```python
from build123d import *

# Parameters (mm, degrees)
SKETCH_1_R      = 1.55
EXTRUDE_1_DEPTH = 3
FILLET_1_R      = 2


with BuildPart() as part:
    # 草图1 → 凸台-拉伸1 (new body)
    with BuildSketch(Plane(origin=(0, 0, 0), x_dir=(0, 0, -1), z_dir=(1, 0, 0))):
        with BuildLine():
            Line((0, 25.4), (0, 0))
            Line((0, 0), (17, 0))
            Line((17, 0), (17, 33))
            Line((17, 33), (-5.5, 33))
            Line((-5.5, 33), (0, 27.5))
            ThreePointArc((0, 27.5), (0.74246212, 27.19246212), (1.05, 26.45))
            ThreePointArc((1.05, 26.45), (0.74246212, 25.70753788), (0, 25.4))
        make_face()
        with Locations((7.75, 5)):
            Circle(SKETCH_1_R, mode=Mode.SUBTRACT)
        with Locations((2.5, 29)):
            Circle(SKETCH_1_R, mode=Mode.SUBTRACT)
        with Locations((7.75, 20)):
            Circle(SKETCH_1_R, mode=Mode.SUBTRACT)
        with Locations((13, 29)):
            Circle(SKETCH_1_R, mode=Mode.SUBTRACT)
    extrude(amount=EXTRUDE_1_DEPTH)

    # 圆角1
    fillet_1_edges = [part.edges().sort_by_distance(p)[0] for p in [
        (1.5, 33, 5.5),
    ]]
    fillet(fillet_1_edges, radius=FILLET_1_R)


solid = part.part
```
The listing builds one solid part. Answer for the finished solid, in the listing's coordinates (mm). A direction names the side the tool comes from. Give positions to 0.01 mm unless a question says otherwise; leave off trailing zeros. Order: outer loops, then holes, each group sorted by start corner. A loop starts at its lowest first (then second) coordinate and runs counter-clockwise, first axis right, second up.
1) Given P1, Ø1.5, axis at x = 0.5, y = 22, coming from the +Z side, flat-ended and moving along its own axis, determine where the tip first touches the part or whether it passes through.
Reported:
P1: stops at z = 0
2) Find section A-A on x = 2.55. Write down the section's boundary in (y, z), then the cut area to 3 significant figures.
Reported:
outline: (0, -17) - (33, -17) - (33, 0.67) arc R2 ccw to (29.59, 2.09) - (27.5, 0) arc R1.05 cw to (25.4, 0) - (0, 0) - close; hole circle Ø3.1 at (5, -7.75); hole circle Ø3.1 at (20, -7.75); hole circle Ø3.1 at (29, -13); hole circle Ø3.1 at (29, -2.5)
area: 539 mm2
3) Find section C-C on y = 5. Write down the section's boundary in (x, z), then the cut area to 3 significant figures.
Reported:
outline: (0, -17) - (3, -17) - (3, -9.3) - (0, -9.3) - close; (0, -6.2) - (3, -6.2) - (3, 0) - (0, 0) - close
area: 41.7 mm2
4) Find section D-D on y = 29. Write down the section's boundary in (x, z), then the cut area to 3 significant figures.
Reported:
outline: (0, -17) - (3, -17) - (3, -14.55) - (0, -14.55) - close; (0, -11.45) - (3, -11.45) - (3, -4.05) - (0, -4.05) - close; (0, -0.95) - (3, -0.95) - (3, 1.5) - (0, 1.5) - close
area: 36.9 mm2
5) For faces 5 (the face through (1, 13, 0)), 6 (the face through (1, 16, -17)), determine the directions among +Z, -Z, +X, -X, +Y, -Y from which every point of the face is accessible in a straight line to the end or side of a thin tool.
Reported:
face 5: +Z, +X, -X, -Y
face 6: -Z, +X, -X, +Y, -Y
6) Find section B-B on z = -7.75. Write down the section's boundary in (x, y).
Reported:
outline: (0, 0) - (3, 0) - (3, 3.45) - (0, 3.45) - close; (0, 6.55) - (3, 6.55) - (3, 18.45) - (0, 18.45) - close; (0, 21.55) - (3, 21.55) - (3, 33) - (0, 33) - close
7) Determine the mould class of faces 1 (the face through (1.479, 5.466, -9.228)), 2 (the face through (1, 33, -8)), 3 (the face through (0, 17, -7)), 4 (the face through (1.5, 28.6, 1.1)) for opening direction Y: pulls with the +Y half, pulls with the -Y half, needs draft (parallel to the pull), parting line crosses it, or undercut.
Reported:
face 1: undercut
face 2: pulls with the +Y half
face 3: needs draft
face 4: pulls with the -Y half
8) Consider line 1 along Y through (x, z) = (2.35, -13); line 2 along Y through (x, z) = (2.35, -9); line 3 along Y through (x, z) = (1.9, -8.5). Determine where each line is inside the solid, lowest interval first.
Reported:
line 1: y = 0 to 27.45, 30.55 to 33
line 2: y = 0 to 4.08, 5.92 to 19.08, 20.92 to 33
line 3: y = 0 to 3.64, 6.36 to 18.64, 21.36 to 33
